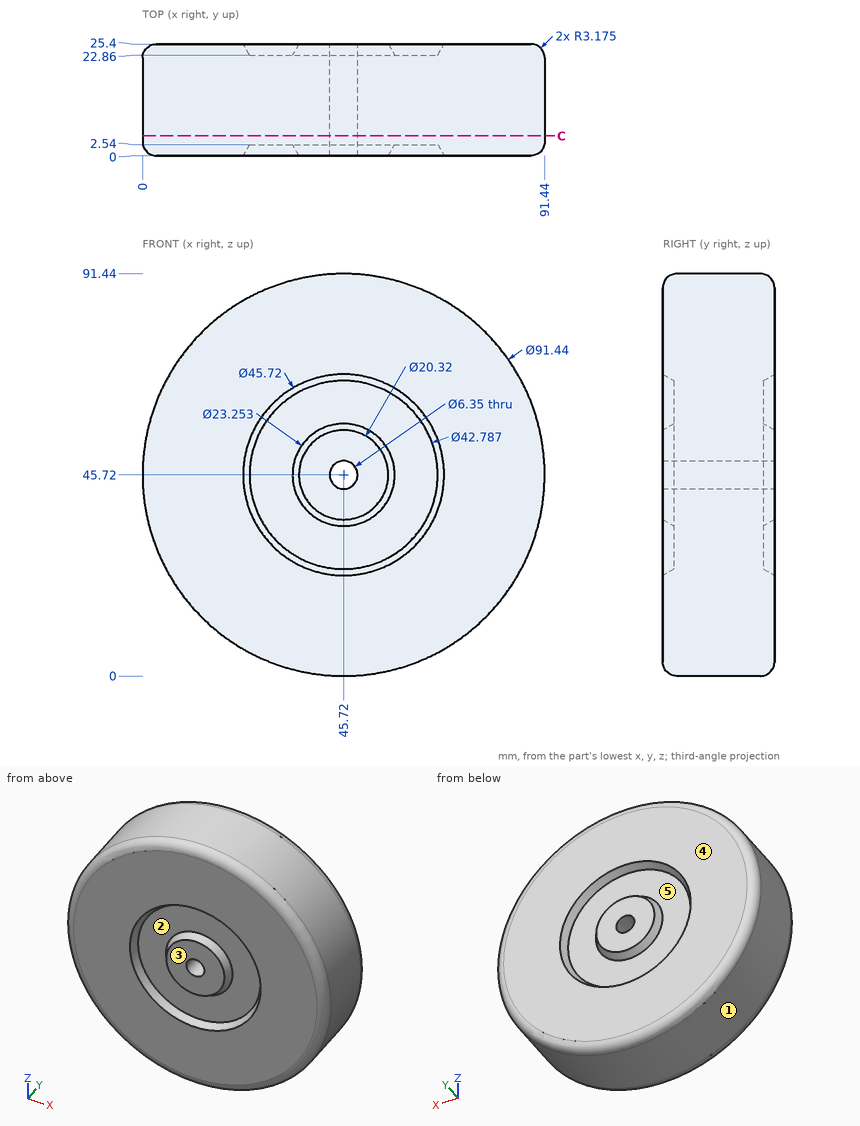
Geometry check sheet. Reference: drawing and pictorial views, mm from the part's lowest x, y, z. A direction names the side the tool comes from. Round coordinates to 2 decimals unless told otherwise and drop trailing zeros. Loops run counter-clockwise (first coordinate to the right, second up) from the corner with the lowest first, then second, coordinate; pieces in that order, holes last.
1. Gauge pin test, flat ends, axial feed: pin 1 Ø10 at (x, z) = (60.5, 37.5) entering from -Y; pin 2 Ø3 at (y, z) = (8, 28) entering from -X; pin 3 Ø1 at (x, z) = (62, 58.5) entering from +Y. Record the tip position at first contact, or that the pin passes through.
2. Scan lines: probe 1 along Z at (x, y) = (45.72, 19.5) (3 decimals); probe 2 along Z at (x, y) = (43, 2). Record each from-to range of solid material in increasing order.
3. Set-up check for the marked faces 4 and 5: record each of +Z, -Z, +X, -X, +Y, -Y from which the full face is reachable in a straight line by a thin tool's end or side.
4. Mould release check, pull along X, two halves, no side actions. Record for the marked faces 1, 2 and 3: released by +X, released by -X, zero draft, split by the parting line, or undercut.
5. Sectioned sample at C-C on y = 4.5. Record the boundary of the cut face in (x, z) (3 decimals), and give its area (3 significant figures).
Recorded:
1. pin 1: stops at y = 1.64
1. pin 2: stops at x = 2.97
1. pin 3: stops at y = 22.86
2. probe 1: z = 0 to 42.545, 48.895 to 91.44
2. probe 2: z = 0.31 to 24.19, 34.74 to 44.08, 47.36 to 56.7, 67.25 to 91.13
3. face 4: +Z, -Z, +X, -X, +Y
3. face 5: +Y
4. face 1: split by the parting line
4. face 2: undercut
4. face 3: zero draft
5. outline: circle Ø91.44 at (45.72, 45.72); hole circle Ø6.35 at (45.72, 45.72)
5. area: 6,540 mm2
